Source: CAD feature listing. Evaluate the final solid. Frame: model axes, mm. Give positions to 0.01 mm unless a question says otherwise; leave off trailing zeros. Order: outer loops, then holes, each group sorted by start corner. A loop starts at its lowest first (then second) coordinate and runs counter-clockwise, first axis right, second up. Notation, with made-up numbers: M -17,87.25 L -1,87.25 A29 cw -1,115.25 Z; hole C 36.25,46.25 d1. An arc over 180 degrees is marked long. Use CSV: the item, a comma, the result in double quotes. Start each with the question number.
Item 1: Section query B-B on z = 2. Return loops of the section in (x, y).
Item 2: Pull-direction query (Z, two-part tool) for faces 1 (the face through (2, 0.3, 3)), 2 (the face through (6.75, 3, 3)), 3 (the face through (0, 3, 6.6)); classes: +Z half, -Z half, draft (parallel to the pull), parting line (faces both ways), or undercut.
Item 3: Section query C-C on y = -3.5. Return loops of the section in (x, z).
Item 4: Section query D-D on x = 2.75. Return loops of the section in (y, z).
Item 5: First-contact query: pin 1 (1 mm diameter, centred on x = 1.5, y = -1.5, fed in from +Z); pin 2 (1.3 mm diameter, centred on x = 1.5, z = 3.5, fed in from -Y); pin 3 (1.2 mm diameter, centred on x = -1, y = -1, fed in from -Z); pin 4 (2 mm diameter, centred on y = -2, z = 2.5, fed in from +X). Flat tips, straight axial feed; report the tip coordinate or a pass-through.
Item 6: Section query A-A on x = -0.25. Return loops of the section in (y, z).
Item 7: Ray query, probe 1 along Y at (x, z) = (5, 3); probe 2 along X at (y, z) = (-1, 2.25); probe 3 along Y at (x, z) = (2, 1.25). Return the intervals inside material, ascending. Write a range as from..to.
from build123d import *

# Parameters (mm, degrees)
SKETCH_W     = 13.5
SKETCH_H     = 6.3
PAD_DEPTH    = 6.6
SKETCH001_W  = 6.5
SKETCH001_H  = 4.2
POCKET_DEPTH = 0.3
SKETCH002_W  = 4.1
SKETCH002_H  = 4
PAD001_DEPTH = 5.3


with BuildPart() as part:
    # Sketch → Pad (new body)
    with BuildSketch(Plane.XY):
        with Locations((0, 3.15)):
            Rectangle(SKETCH_W, SKETCH_H)
    extrude(amount=PAD_DEPTH)

    # Sketch001 (on Face3 of Pad) → Pocket (cut)
    with BuildSketch(Plane.XZ):
        with Locations((0, 3.3)):
            Rectangle(SKETCH001_W, SKETCH001_H)
    extrude(amount=-POCKET_DEPTH, mode=Mode.SUBTRACT)

    # Sketch002 (on Face11 of Pocket) → Pad001 (join)
    with BuildSketch(Plane.XZ.offset(-0.3)):
        with Locations((-1.1, 3.3)):
            Rectangle(SKETCH002_W, SKETCH002_H)
    extrude(amount=PAD001_DEPTH)


solid = part.part
Verdict:
1,outline,"M -6.75,0 L -3.25,0 L -3.25,0.3 L -3.15,0.3 L -3.15,-5 L 0.95,-5 L 0.95,0.3 L 3.25,0.3 L 3.25,0 L 6.75,0 L 6.75,6.3 L -6.75,6.3 Z"
2,face 1,"undercut"
2,face 2,"draft"
2,face 3,"+Z half"
3,outline,"M -3.15,1.3 L 0.95,1.3 L 0.95,5.3 L -3.15,5.3 Z"
4,outline,"M 0,0 L 6.3,0 L 6.3,6.6 L 0,6.6 L 0,5.4 L 0.3,5.4 L 0.3,1.2 L 0,1.2 Z"
5,pin 1,"through"
5,pin 2,"y = -5"
5,pin 3,"z = 1.3"
5,pin 4,"x = 0.95"
6,outline,"M -5,1.3 L 0.3,1.3 L 0.3,1.2 L 0,1.2 L 0,0 L 6.3,0 L 6.3,6.6 L 0,6.6 L 0,5.4 L 0.3,5.4 L 0.3,5.3 L -5,5.3 Z"
7,probe 1,"0..6.3"
7,probe 2,"-3.15..0.95"
7,probe 3,"0.3..6.3"
